Verification items for the finished model (mm, model axes). A direction names the side the tool comes from. Coordinates: 2 decimals unless noted, no trailing zeros. Write each loop counter-clockwise with the first axis right and the second up, starting at its lowest first coordinate (ties: lowest second). Pieces come first, ordered by that corner, then holes. Notation, with made-up numbers: (54.25, 58) -> (102.25, 58) arc R25 cw to (102.25, 84) -> close; hole circle Ø7 at (57.5, 34.25). An arc over 180 degrees is marked (long way). Use CSV: the item, a comma, the result in double quotes.
```python
from build123d import *

# Parameters (mm, degrees)
F0_W     = 50
F0_H     = 50
F1_DEPTH = 40
F2_SIZE  = 6
F3_W     = 83.7730430067
F3_H     = 50.7384873927
F4_DEPTH = 25


with BuildPart() as f1:
    # F0 (on Top) → F1 (new body)
    with BuildSketch(Plane.XY):
        Rectangle(F0_W, F0_H)
    extrude(amount=F1_DEPTH)

    # F2
    f2_edges = [f1.edges().sort_by_distance(p)[0] for p in [
        (0, -25, 40),
        (25, 0, 40),
        (0, 25, 40),
        (-25, 0, 40),
        (25, -25, 20),
        (25, 25, 20),
        (-25, -25, 20),
        (-25, 25, 20),
    ]]
    chamfer(f2_edges, length=F2_SIZE)

    # F3 (on Right) → F4 (cut)
    with BuildSketch(Plane.YZ):
        with Locations((1.3156887144, 25.3692436963)):
            Rectangle(F3_W, F3_H)
    extrude(amount=F4_DEPTH, mode=Mode.SUBTRACT)

    # F5 (on face) → F6 (revolve, cut)
    with BuildSketch(Plane.YZ):
        with BuildLine():
            add(Edge.make_bspline(
                [(0, 8.81283544), (-7.6750135049, 8.8968714699), (-15.6428759777, 7.7376163766), (-21.3710906151, 12.9309668683), (-21.3286430979, 20.6974018657), (-20.5851575354, 29.1049836415), (-20.0912714693, 32.8565548223), (-15.8713216928, 36.1712388493), (-10.2699402926, 36.5207207773), (-5.8143442687, 37.0119311275), (-3.7, 37.1318450321)],
                knots=[0, 0, 0, 0, 0.1841228893, 0.2950075682, 0.4215719078, 0.5555240151, 0.642229878, 0.7414659734, 0.8575719069, 0.9488735314, 0.9488735314, 0.9488735314, 0.9488735314], degree=3))
            Line((0, 8.81283544), (0, 37.2170992196))
            add(Edge.make_bspline(
                [(-3.7, 37.1318450321), (-2.5160237402, 37.1989936126), (-1.2840796224, 37.235939493), (0, 37.2170992196)],
                knots=[0.9488735314, 0.9488735314, 0.9488735314, 0.9488735314, 1, 1, 1, 1], degree=3))
        make_face()
        with BuildLine():
            Line((-3.7, 40), (-3.7, 37.1318450321))
            add(Edge.make_bspline(
                [(-3.7, 37.1318450321), (-2.5160237402, 37.1989936126), (-1.2840796224, 37.235939493), (0, 37.2170992196)],
                knots=[0.9488735314, 0.9488735314, 0.9488735314, 0.9488735314, 1, 1, 1, 1], degree=3))
            Line((0, 37.2170992196), (0, 40))
            Line((0, 40), (-3.7, 40))
        make_face()
    revolve(axis=Axis((0, 0, 24.40641772), (0, 0, -1)), mode=Mode.SUBTRACT)


solid = f1.part
```
1) Set-up check for faces 1 (the flat face through (-22, 0, 37)), 2 (the cylindrical face through (-3.7, -0.1, 38.5)): record each of +Z, -Z, +X, -X, +Y, -Y from which the full face is reachable in a straight line by a thin tool's end or side.
Return value:
face 1,"+Z, -X, +Y, -Y"
face 2,"+Z, +X"
2) Cross-section at B-B (x = -23). Record the boundary of the cut face in (y, z), plus the area to 3 significant figures.
Return value:
outline,"(-21, 0) -> (21, 0) -> (21, 34) -> (19, 36) -> (-19, 36) -> (-21, 34) -> close"
area,"1,510 mm2"
3) Scan lines: L1, parallel to Y at x = -17, z = 15; L2, parallel to Z at x = -4, y = 9.5; L3, parallel to Y at x = -5.25, z = 33. Record each from-to range of solid material in increasing order.
Return value:
L1,"-25 to -12.34, 12.34 to 25"
L2,"0 to 8.66, 36.57 to 40"
L3,"-25 to -18.66, 18.66 to 25"
4) Cross-section at A-A (z = 4). Record the boundary of the cut face in (x, y), plus the area to 3 significant figures.
Return value:
outline,"(-25, -19) -> (-19, -25) -> (0, -25) -> (0, 25) -> (-19, 25) -> (-25, 19) -> close"
area,"1,210 mm2"
